Part model, mm, in its own coordinate system. Round coordinates to 2 decimals unless told otherwise and drop trailing zeros. Write each loop counter-clockwise with the first axis right and the second up, starting at its lowest first coordinate (ties: lowest second). Pieces come first, ordered by that corner, then holes.
```python
from build123d import *

# Parameters (mm, degrees)
F1_R     = 10
F1_R_2   = 5
F2_DEPTH = 18
F3_DEPTH = 12


with BuildPart() as f2:
    # F1 (on Front) → F2 (new body)
    with BuildSketch(Plane.XZ):
        with BuildLine():
            Line((-400, 0), (0, 0))
            Line((0, 0), (400, 0))
            Line((400, 0), (400, 50))
            ThreePointArc((400, 50), (385.3553390593, 85.3553390593), (350, 100))
            Line((350, 100), (245.256839525, 100))
            ThreePointArc((245.256839525, 100), (211.7035324399, 112.9301256591), (195.5041644303, 145.032976654))
            Line((195.5041644303, 145.032976654), (49.7526750947, 1604.967023346))
            ThreePointArc((49.7526750947, 1604.967023346), (0, 1650), (-49.7526750947, 1604.967023346))
            Line((-49.7526750947, 1604.967023346), (-195.5041644303, 145.032976654))
            ThreePointArc((-195.5041644303, 145.032976654), (-211.7035324399, 112.9301256591), (-245.256839525, 100))
            Line((-245.256839525, 100), (-350, 100))
            ThreePointArc((-350, 100), (-385.3553390593, 85.3553390593), (-400, 50))
            Line((-400, 50), (-400, 0))
        make_face()
        with Locations((-250, 50)):
            Circle(F1_R, mode=Mode.SUBTRACT)
        with Locations((250, 50)):
            Circle(F1_R, mode=Mode.SUBTRACT)
        with Locations((0, 1600)):
            Circle(F1_R, mode=Mode.SUBTRACT)
        with Locations((0, 1600)):
            Circle(F1_R)
        with Locations((0, 1600)):
            Circle(F1_R_2, mode=Mode.SUBTRACT)
        with Locations((-250, 50)):
            Circle(F1_R)
        with Locations((-250, 50)):
            Circle(F1_R_2, mode=Mode.SUBTRACT)
        with Locations((250, 50)):
            Circle(F1_R)
        with Locations((250, 50)):
            Circle(F1_R_2, mode=Mode.SUBTRACT)
    extrude(amount=F2_DEPTH)

    # F1 (on Front) → F3 (cut)
    with BuildSketch(Plane.XZ):
        with Locations((0, 1600)):
            Circle(F1_R)
        with Locations((0, 1600)):
            Circle(F1_R_2, mode=Mode.SUBTRACT)
        with Locations((250, 50)):
            Circle(F1_R)
        with Locations((250, 50)):
            Circle(F1_R_2, mode=Mode.SUBTRACT)
        with Locations((-250, 50)):
            Circle(F1_R)
        with Locations((-250, 50)):
            Circle(F1_R_2, mode=Mode.SUBTRACT)
    extrude(amount=F3_DEPTH, mode=Mode.SUBTRACT)


solid = f2.part
```
Q1. Drop flat-ended pins along their axis: pin 1 (2 mm diameter, centred on x = -1, y = -8.5, fed in from +Z); pin 2 (10 mm diameter, centred on x = 253, z = 52.5, fed in from +Y); pin 3 (10 mm diameter, centred on x = 315.5, y = -14.5, fed in from +Z). Give the stop position or say it passes through.
Values follow:
pin 1: stops at z = 1650
pin 2: stops at y = -12
pin 3: stops at z = 100
Q2. Cut at B-B on x = 280.5. Write the cut outline in (y, z).
Values follow:
outline: (-18, 0) - (0, 0) - (0, 100) - (-18, 100) - close
Q3. Cut at A-A on y = -4.25. Write the cut outline in (x, z), plus the area to 3 significant figures.
Values follow:
outline: (-400, 0) - (400, 0) - (400, 50) arc R50 ccw to (350, 100) - (245.26, 100) arc R50 cw to (195.5, 145.03) - (49.75, 1604.97) arc R50 ccw to (-49.75, 1604.97) - (-195.5, 145.03) arc R50 cw to (-245.26, 100) - (-350, 100) arc R50 ccw to (-400, 50) - close; hole circle Ø20 at (-250, 50); hole circle Ø20 at (0, 1600); hole circle Ø20 at (250, 50)
area: 458,000 mm2
Q4. Cut at C-C on z = 1413.5. Write the cut outline in (x, y).
Values follow:
outline: (-68.87, -18) - (68.87, -18) - (68.87, 0) - (-68.87, 0) - close
Q5. Wall check: L1, parallel to Z at x = 250, y = -3.5; L2, parallel to Z at x = -250, y = -13.9; L3, parallel to Z at x = -313.5, y = -0.75. Give the ranges that are in metal, low to high.
Values follow:
L1: z = 0 to 40, 60 to 100
L2: z = 0 to 45, 55 to 100
L3: z = 0 to 100
